For this review, take the finished solid that the model builds, in its own axes (mm). A direction names the side the tool comes from. Coordinates: 2 decimals unless noted, no trailing zeros. Order: outer loops, then holes, each group sorted by start corner. A loop starts at its lowest first (then second) coordinate and runs counter-clockwise, first axis right, second up. Notation, with made-up numbers: (3.25, -25.75) - (20.25, -25.75) arc R19 cw to (20.25, -8.75) - close; hole circle Ø10 at (88, 6.25). An arc over 180 degrees is marked (long way). One line per item, written item: value. Start each with the question number.
(1) Consider section C-C on y = -7.25. Write out the cut boundary in (x, z).
(2) Consider section B-B on z = -28.5. Write out the cut boundary in (x, y), then the cut area to 3 significant figures.
(3) Consider section D-D on z = -64.5. Write out the cut boundary in (x, y).
(4) Mouldability with a two-part tool opening along Z and no side actions: class faces 1 (the flat face through (36.977, -20.563, -25.947)), 2 (the flat face through (38, -12, -8)), 3 (the flat face through (-26.196, -12.675, -56.054)) as released by +Z, released by -Z, zero draft, split by the parting line, or undercut.
(5) To check wall thickness, follow line 1 along X through (y, z) = (-13.5, -15.5); line 2 along X through (y, z) = (-5.5, -6.5); line 3 along X through (y, z) = (-24, 70). State the ranges of each line that lie inside material, in increasing order.
(6) For faces 4 (the flat face through (40, -12, 0)), 5 (the flat face through (0, -12, -8)), 6 (the flat face through (17, -12, -44)), 7 (the flat face through (19.231, -4.563, -34.465)), list the 3-axis set-ups (+Z, -Z, +X, -X, +Y, -Y) from which the entire face can be reached by the end or side of a thin tool; tool diameter is ignored.
(7) Consider section A-A on x = -16.5. Write out the cut boundary in (y, z), then the cut area to 3 significant figures.
(8) Clearance check with flat-ended pins moving along their axes: pin 1 (12 mm diameter, centred on y = -19, z = 80.5, fed in from +X); pin 2 (4.5 mm diameter, centred on x = 39.5, y = -10, fed in from +Z); pin 3 (12.5 mm diameter, centred on x = 15.5, y = -10, fed in from -Z). State where each tip first meets the part, or that it passes through.
```python
from build123d import *

# Parameters (mm, degrees)
F1_DEPTH = 25
F2_SIZE2 = 5
F2_SIZE  = 9
F3_SIZE2 = 9
F3_SIZE  = 5
F4_R     = 8
F5_R     = 12.49999
F6_SIZE2 = 39.99999
F6_SIZE  = 59.99999
F7_SIZE  = 39.99999
F9_DEPTH = 25.001


# Not quite as in the source:
# - a fillet or chamfer is up to 0.001 mm smaller than in the source, because OpenCascade refuses the exact size


with BuildPart() as f1:
    # F0 (on Front) → F1 (new body)
    with BuildSketch(Plane.XZ):
        Polygon((0, -16), (0, 0), (-40, 0), (-40, 100), (-50, 100), (-50, -84), (-40, -84), (-40, -44), (40.316005618, -44), (50, -18.1760149813), (50, 0), (38, 0), (38, -16), (32, -32), (6, -32), align=None)
    extrude(amount=F1_DEPTH)

    # F2
    f2_edges = [f1.edges().sort_by_distance(p)[0] for p in [
        (19, -25, -32),
        (3, -25, -24),
        (0, -25, -8),
        (35, -25, -24),
        (38, -25, -8),
    ]]
    chamfer(f2_edges, length=F2_SIZE, length2=F2_SIZE2)

    # F3
    f3_edges = [f1.edges().sort_by_distance(p)[0] for p in [
        (19, 0, -32),
        (3, 0, -24),
        (0, 0, -8),
        (35, 0, -24),
        (38, 0, -8),
    ]]
    f3_side = f1.faces().sort_by_distance((-19.786858, 0, -11.21384))[0]
    chamfer(f3_edges, length=F3_SIZE, length2=F3_SIZE2, reference=f3_side)

    # F4
    f4_edges = [f1.edges().sort_by_distance(p)[0] for p in [
        (40.316006, -12.5, -44),
        (50, -12.5, -18.176015),
        (50, -12.5, 0),
    ]]
    fillet(f4_edges, radius=F4_R)

    # F5 (radius 12.5 in the source; OpenCascade refuses exactly that, so slightly less here)
    f5_edges = [f1.edges().sort_by_distance(p)[0] for p in [
        (-45, -25, -84),
        (-45, 0, -84),
        (-45, -25, 100),
        (-45, 0, 100),
    ]]
    fillet(f5_edges, radius=F5_R)

    # F6 (size 60 and 40 in the source; OpenCascade refuses exactly that, so slightly less here)
    f6_edges = [f1.edges().sort_by_distance(p)[0] for p in [
        (-40, -12.5, 0),
    ]]
    f6_side = f1.faces().sort_by_distance((-40, -12.5, 48.698732))[0]
    chamfer(f6_edges, length=F6_SIZE, length2=F6_SIZE2, reference=f6_side)

    # F7 (size 40 in the source; OpenCascade refuses exactly that, so slightly less here)
    f7_edges = [f1.edges().sort_by_distance(p)[0] for p in [
        (-40, -12.5, -44),
    ]]
    chamfer(f7_edges, length=F7_SIZE)

    # F8 (on face) → F9 (cut, through all)
    with BuildSketch(Plane.XZ.offset(25)):
        Polygon((-12, -0.0277563773), (-40, 41.9722436227), (-40, -69.8578643763), (-12, -41.8578643763), align=None)
    extrude(amount=-F9_DEPTH, mode=Mode.SUBTRACT)


solid = f1.part
```
Geometry check:
1. outline: (-50, -82.84) - (-38.84, -82.84) - (0, -44) - (34.77, -44) arc R8 ccw to (42.26, -38.81) - (49.49, -19.53) arc R8 ccw to (50, -16.73) - (50, -8) arc R8 ccw to (42, 0) - (38.97, 0) - (38.97, -16.18) - (32.67, -32.97) - (5.33, -32.97) - (-0.97, -16.18) - (-0.97, 1.46) - (-40, 60) - (-40, 98.84) - (-50, 98.84) - close; hole (-40, -69.86) - (-12, -41.86) - (-12, -0.03) - (-40, 41.97) - close
2. outline: (-50, -25) - (-40, -25) - (-40, 0) - (-50, 0) - close; (-12, -25) - (-0.65, -25) - (4.69, -16) - (4.69, -9) - (-0.65, 0) - (-12, 0) - close; (33.31, -16) - (38.65, -25) - (46.13, -25) - (46.13, 0) - (38.65, 0) - (33.31, -9) - close
2. area: 891 mm^2
3. outline: (-50, -25) - (-40, -25) - (-40, 0) - (-50, 0) - close; (-34.64, -25) - (-20.5, -25) - (-20.5, 0) - (-34.64, 0) - close
4. face 1: released by +Z
4. face 2: zero draft
4. face 3: undercut
5. line 1: x = -50 to -40, -12 to 0, 38 to 50
5. line 2: x = -50 to -40, -12 to -1.94, 39.94 to 49.86
5. line 3: x = -50 to -40
6. face 4: +Z, +X, +Y, -Y
6. face 5: +Z, +Y, -Y
6. face 6: -Z, +X, +Y, -Y
6. face 7: +Z, +Y
7. outline: (-25, -60.5) - (0, -60.5) - (0, -46.36) - (-25, -46.36) - close; (-25, 6.72) - (0, 6.72) - (0, 24.75) - (-25, 24.75) - close
7. area: 804 mm^2
8. pin 1: stops at x = -40
8. pin 2: stops at z = 0
8. pin 3: stops at z = -44
